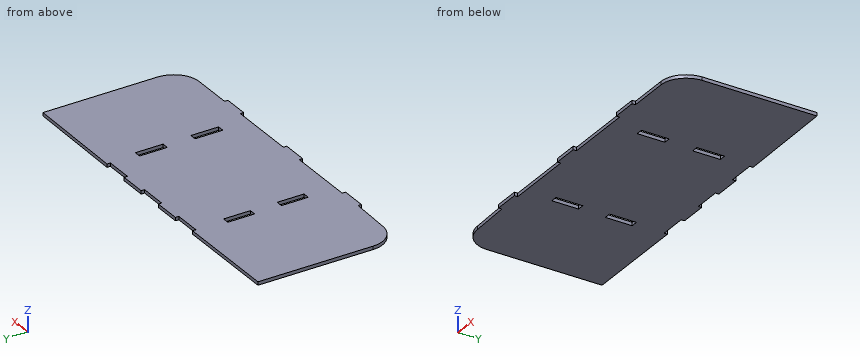
from build123d import *

# Parameters (mm, degrees)
SKETCH1_W           = 20.32
SKETCH1_H           = 81.316938585
SKETCH1_H_2         = 84.113540858
BOSS_EXTRUDE1_DEPTH = 10.16


with BuildPart() as part:
    # Sketch1 → Boss-Extrude1 (new body)
    # profile 1 of 2: a face of its own
    with BuildSketch(Plane.XY):
        with BuildLine():
            ThreePointArc((-520.699999986, 86.36), (-498.381536717, 32.478463279), (-444.5, 10.16))
            Line((-444.5, 10.16), (-321.2, 6.224098454))
            Line((-321.2, 6.224098454), (-321.2, -3.935901546))
            Line((-321.2, -3.935901546), (-245, -3.935901546))
            Line((-245, -3.935901546), (-245, 6.224098454))
            Line((-245, 6.224098454), (-38.1, 6.224098454))
            Line((-38.1, 6.224098454), (-38.1, -3.935901546))
            Line((-38.1, -3.935901546), (38.1, -3.935901546))
            Line((38.1, -3.935901546), (38.1, 6.224098454))
            Line((38.1, 6.224098454), (245, 6.224098454))
            Line((245, 6.224098454), (245, -3.935901546))
            Line((245, -3.935901546), (321.2, -3.935901546))
            Line((321.2, -3.935901546), (321.2, 6.224098454))
            Line((321.2, 6.224098454), (444.500003861, 6.224098454))
            add(Edge.make_bspline(
                [(444.500003861, 6.224098454), (516.375223264, 6.870661069), (520.046520409, 82.264098454)],
                knots=[3.150157412, 3.150157412, 3.150157412, 4.661289858, 4.661289858, 4.661289858], degree=2, weights=[1, 0.7278834, 1]))
            Line((520.046520409, 82.264098454), (520.070316171, 431.514078957))
            Line((520.070316171, 431.514078957), (205.706405146, 435.61))
            Line((205.706405146, 435.61), (205.558012439, 425.45))
            Line((205.558012439, 425.45), (123.444, 425.45))
            Line((123.444, 425.45), (123.444, 435.61))
            Line((123.444, 435.61), (41.148, 435.61))
            Line((41.148, 435.61), (41.148, 425.45))
            Line((41.148, 425.45), (-41.148, 425.45))
            Line((-41.148, 425.45), (-41.148, 435.61))
            Line((-41.148, 435.61), (-123.444, 435.61))
            Line((-123.444, 435.61), (-123.444, 425.45))
            Line((-123.444, 425.45), (-205.739999986, 425.45))
            Line((-205.739999986, 425.45), (-205.739999986, 388.35))
            Line((-205.739999986, 388.35), (-230.359692704, 388.35))
            Line((-230.359692704, 388.35), (-230.359692704, 435.61))
            Line((-230.359692704, 435.61), (-520.3601107, 435.61))
            Line((-520.3601107, 435.61), (-520.699999986, 86.36))
        make_face()
        with Locations((-206.375268781, 132.135407878)):
            Rectangle(SKETCH1_W, SKETCH1_H, mode=Mode.SUBTRACT)
        with Locations((206.375268781, 132.394409741)):
            Rectangle(SKETCH1_W, SKETCH1_H_2, mode=Mode.SUBTRACT)
        with Locations((-206.375268781, 294.769285048)):
            Rectangle(SKETCH1_W, SKETCH1_H, mode=Mode.SUBTRACT)
        with Locations((206.375268781, 300.621491457)):
            Rectangle(SKETCH1_W, SKETCH1_H_2, mode=Mode.SUBTRACT)
    # profile 2 of 2: a face of its own
    with BuildSketch(Plane.XY):
        Polygon((-205.739999986, 435.61), (-230.359692704, 435.61), (-230.359692704, 388.35), (-205.739999986, 388.35), (-205.739999986, 425.45), align=None)
    extrude(amount=BOSS_EXTRUDE1_DEPTH)


solid = part.part
Could you check a few things on this model? Use its own coordinates, in mm. Give positions to 0.01 mm unless a question says otherwise; leave off trailing zeros. Order: outer loops, then holes, each group sorted by start corner. A loop starts at its lowest first (then second) coordinate and runs counter-clockwise, first axis right, second up.
1. Suppose I cut it at B-B (x = -3). List the corners of the cut face in (y, z) for me, plus the area to 3 significant figures.
2. Suppose I cut it at A-A (y = 274). List the corners of the cut face in (x, z) for me, plus the area to 3 significant figures.
3. I need wall thicknesses on L1, parallel to Y at x = 209.5, z = 0.75; L2, parallel to X at y = 316, z = 3.25; L3, parallel to X at y = 212, z = 5. Which ranges of each line are inside material? Lowest first, please.
4. Suppose I cut it at C-C (z = 6.25). Give the number of separate pieces and of enclosed holes in the cut face, plus the area to 3 significant figures.
5. Will these pins go through, and if not, where does the flat tip stop? P1, Ø4, axis at x = 336.5, z = 8, coming from the +Y side; P2, Ø3, axis at y = 3, z = 3, coming from the -X side; P3, Ø4, axis at y = 195.5, z = 5, coming from the +X side.
6. Suppose I cut it at D-D (x = 157.5). List the corners of the cut face in (y, z) for me.
Solved:
1. outline: (-3.94, 0) - (425.45, 0) - (425.45, 10.16) - (-3.94, 10.16) - close
1. area: 4,360 mm2
2. outline: (-520.52, 0) - (-216.54, 0) - (-216.54, 10.16) - (-520.52, 10.16) - close; (-196.22, 0) - (196.22, 0) - (196.22, 10.16) - (-196.22, 10.16) - close; (216.54, 0) - (520.06, 0) - (520.06, 10.16) - (216.54, 10.16) - close
2. area: 10,200 mm2
3. L1: y = 6.22 to 90.34, 174.45 to 258.56, 342.68 to 435.56
3. L2: x = -520.48 to -216.54, -196.22 to 196.22, 216.54 to 520.06
3. L3: x = -520.58 to 520.06
4. separate pieces: 1
4. enclosed holes: 4
4. area: 436,000 mm2
5. P1: stops at y = 433.93
5. P2: stops at x = -321.2
5. P3: stops at x = 520.05
6. outline: (6.22, 0) - (425.45, 0) - (425.45, 10.16) - (6.22, 10.16) - close
